Can you work these out from the model? Positions are in its coordinate system, mm. Face numbers are marked on the shaded views. Round coordinates to 2 decimals unless told otherwise and drop trailing zeros. Loops run counter-clockwise (first coordinate to the right, second up) from the corner with the lowest first, then second, coordinate; pieces in that order, holes last. Notation, with made-up numbers: M -2.75,-35 L 39.25,-35 A11 cw 39.25,-23 Z; hole C -8,45.25 d11. An arc over 180 degrees is marked long. Use a Markdown table: item, result. Add a question column.
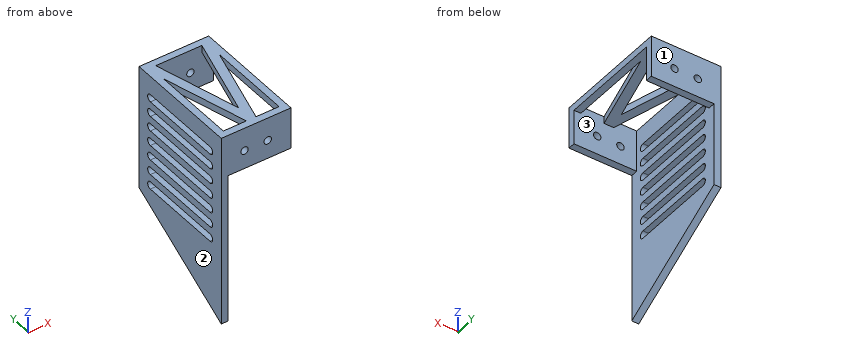
```python
from build123d import *

# Parameters (mm, degrees)
SKETCH_1_W      = 30
SKETCH_1_H      = 50
EXTRUDE_1_DEPTH = 3
EXTRUDE_3_DEPTH = 3
EXTRUDE_START   = -50
SKETCH_3_W      = 27
SKETCH_3_H      = 15
SKETCH_3_R      = 1.6
EXTRUDE_4_DEPTH = 3
SKETCH_5_W      = 27
SKETCH_5_H      = 15
SKETCH_5_R      = 1.6
EXTRUDE_5_DEPTH = 3


with BuildPart() as part:
    # 草图1 → 凸台-拉伸1 (new body)
    with BuildSketch(Plane.XY):
        with Locations((-1.547723223, -1.182673383)):
            Rectangle(SKETCH_1_W, SKETCH_1_H)
        Polygon((-13.547723223, 13.216157116), (-13.547723223, -23.182673383), (-3.620769451, -23.182673383), align=None, mode=Mode.SUBTRACT)
        Polygon((10.452276777, 13.216157116), (10.452276777, -23.182673383), (0.525323004, -23.182673383), align=None, mode=Mode.SUBTRACT)
        Polygon((-11.474676996, 20.817326617), (8.379230549, 20.817326617), (-1.547723223, -15.581503883), align=None, mode=Mode.SUBTRACT)
    extrude(amount=EXTRUDE_1_DEPTH)

    # 草图2 → 凸台-拉伸3 (add)
    with BuildSketch(Plane.ZY.offset(16.547723223)):
        Polygon((-80, -26.182673383), (-51.132486541, 23.817326617), (0, 23.817326617), (0, -26.182673383), align=None)
        Polygon((-3, -23.182673383), (-3, 20.817326617), (-49.400435733, 20.817326617), (-74.803847577, -23.182673383), align=None, mode=Mode.SUBTRACT)
        Polygon((-3, -23.182673383), (-74.803847577, -23.182673383), (-49.400435733, 20.817326617), (-3, 20.817326617), align=None)
        with BuildLine():
            ThreePointArc((-8.378224309, -19.337056165), (-6.74645341, -20.968827063), (-5.114682512, -19.337056165))
            Line((-5.114682512, -19.337056165), (-5.114682512, 16.93515829))
            ThreePointArc((-5.114682512, 16.93515829), (-6.74645341, 18.566929189), (-8.378224309, 16.93515829))
            Line((-8.378224309, 16.93515829), (-8.378224309, -19.337056165))
        make_face(mode=Mode.SUBTRACT)
        with BuildLine():
            ThreePointArc((-14.878224309, -19.337056165), (-13.24645341, -20.968827063), (-11.614682512, -19.337056165))
            Line((-11.614682512, -19.337056165), (-11.614682512, 16.93515829))
            ThreePointArc((-11.614682512, 16.93515829), (-13.24645341, 18.566929189), (-14.878224309, 16.93515829))
            Line((-14.878224309, 16.93515829), (-14.878224309, -19.337056165))
        make_face(mode=Mode.SUBTRACT)
        with BuildLine():
            ThreePointArc((-21.378224309, -19.337056165), (-19.74645341, -20.968827063), (-18.114682512, -19.337056165))
            Line((-18.114682512, -19.337056165), (-18.114682512, 16.93515829))
            ThreePointArc((-18.114682512, 16.93515829), (-19.74645341, 18.566929189), (-21.378224309, 16.93515829))
            Line((-21.378224309, 16.93515829), (-21.378224309, -19.337056165))
        make_face(mode=Mode.SUBTRACT)
        with BuildLine():
            ThreePointArc((-27.878224309, -19.337056165), (-26.24645341, -20.968827063), (-24.614682512, -19.337056165))
            Line((-24.614682512, -19.337056165), (-24.614682512, 16.93515829))
            ThreePointArc((-24.614682512, 16.93515829), (-26.24645341, 18.566929189), (-27.878224309, 16.93515829))
            Line((-27.878224309, 16.93515829), (-27.878224309, -19.337056165))
        make_face(mode=Mode.SUBTRACT)
        with BuildLine():
            ThreePointArc((-34.378224309, -19.337056165), (-32.74645341, -20.968827063), (-31.114682512, -19.337056165))
            Line((-31.114682512, -19.337056165), (-31.114682512, 16.93515829))
            ThreePointArc((-31.114682512, 16.93515829), (-32.74645341, 18.566929189), (-34.378224309, 16.93515829))
            Line((-34.378224309, 16.93515829), (-34.378224309, -19.337056165))
        make_face(mode=Mode.SUBTRACT)
        with BuildLine():
            ThreePointArc((-40.878224309, -19.337056165), (-39.24645341, -20.968827063), (-37.614682512, -19.337056165))
            Line((-37.614682512, -19.337056165), (-37.614682512, 16.93515829))
            ThreePointArc((-37.614682512, 16.93515829), (-39.24645341, 18.566929189), (-40.878224309, 16.93515829))
            Line((-40.878224309, 16.93515829), (-40.878224309, -19.337056165))
        make_face(mode=Mode.SUBTRACT)
        with BuildLine():
            ThreePointArc((-47.378224309, -19.337056165), (-45.74645341, -20.968827063), (-44.114682512, -19.337056165))
            Line((-44.114682512, -19.337056165), (-44.114682512, 16.93515829))
            ThreePointArc((-44.114682512, 16.93515829), (-45.74645341, 18.566929189), (-47.378224309, 16.93515829))
            Line((-47.378224309, 16.93515829), (-47.378224309, -19.337056165))
        make_face(mode=Mode.SUBTRACT)
    extrude(amount=-EXTRUDE_3_DEPTH)

    # 草图3 → 凸台-拉伸4 (add)
    with BuildSketch(Plane(origin=(0, 23.817326617, 0), x_dir=(1, 0, 0), z_dir=(0, 1, 0)).offset(EXTRUDE_START)):
        with Locations((-0.047723223, 7.5)):
            Rectangle(SKETCH_3_W, SKETCH_3_H)
        with Locations((-6.547723223, 7)):
            Circle(SKETCH_3_R, mode=Mode.SUBTRACT)
        with Locations((3.452276777, 7)):
            Circle(SKETCH_3_R, mode=Mode.SUBTRACT)
    extrude(amount=EXTRUDE_4_DEPTH)

    # 草图5 → 凸台-拉伸5 (add)
    with BuildSketch(Plane(origin=(0, 23.817326617, 0), x_dir=(1, 0, 0), z_dir=(0, 1, 0))):
        with Locations((-0.047723223, 7.5)):
            Rectangle(SKETCH_5_W, SKETCH_5_H)
        with Locations((-6.547723223, 7)):
            Circle(SKETCH_5_R, mode=Mode.SUBTRACT)
        with Locations((3.452276777, 7)):
            Circle(SKETCH_5_R, mode=Mode.SUBTRACT)
    extrude(amount=-EXTRUDE_5_DEPTH)


solid = part.part
```
(1) Thinking about a two-plate mould opening in Y: for the marked faces 1, 2 and 3, which applies, released by +Y, released by -Y, zero draft, split by the parting line, or undercut?
(2) Suppose I cut it at A-A on z = -39. List the corners of the cut face in (x, y) for me, and give its area (3 significant figures).
(3) I'm going to push flat-ended pins straight in: pin 1 (0.9 mm diameter, centred on x = -15, y = -2.5, fed in from -Z); pin 2 (4 mm diameter, centred on y = -20, z = -9.5, fed in from +X); pin 3 (3.5 mm diameter, centred on x = -15, y = -1, fed in from -Z). Where does each tip first touch, or does it pass through?
(4) If I drill on probe 1 along X at (y, z) = (22.25, -7); probe 2 along Y at (x, z) = (-5, -8.5); probe 3 along X at (y, z) = (-17.5, -44), over which ranges is the centre line in solid material (lowest first)? Write a range as [from, to].
(5) Suppose I cut it at D-D on y = -11.5. Count the separate pieces of the cut face and the enclosed holes in it, and give its area (3 significant figures).
(6) Suppose I cut it at C-C on x = 2.75. List the corners of the cut face in (y, z) for me.
(7) Suppose I cut it at B-B on z = -7. List the corners of the cut face in (x, y) for me, and give its area (3 significant figures).
Results below:
| question | item | result |
|---|---|---|
| 1 | face 1 | released by +Y |
| 1 | face 2 | zero draft |
| 1 | face 3 | undercut |
| 2 | outline | M -16.55,-26.18 L -13.55,-26.18 L -13.55,-20.95 L -16.55,-20.95 Z; M -16.55,18.55 L -13.55,18.55 L -13.55,23.82 L -16.55,23.82 Z |
| 2 | area | 31.5 mm² |
| 3 | pin 1 | stops at z = -66.59 |
| 3 | pin 2 | stops at x = -13.55 |
| 3 | pin 3 | stops at z = -66.47 |
| 4 | probe 1 | x = [-16.55, -8.15], [-4.95, 1.85], [5.05, 13.45] |
| 4 | probe 2 | y = [-26.18, -23.18], [20.82, 23.82] |
| 4 | probe 3 | x = [-16.55, -13.55] |
| 5 | separate pieces | 11 |
| 5 | enclosed holes | 0 |
| 5 | area | 189 mm² |
| 6 | outline | M -26.18,-15 L -23.18,-15 L -23.18,-8.44 L -26.18,-8.44 Z; M -26.18,-5.56 L -23.18,-5.56 L -23.18,3 L -26.18,3 Z; M -15.03,0 L 0.18,0 L 0.18,3 L -15.03,3 Z; M 20.82,-15 L 23.82,-15 L 23.82,-8.44 L 20.82,-8.44 Z; M 20.82,-5.56 L 23.82,-5.56 L 23.82,3 L 20.82,3 Z |
| 7 | outline | M -16.55,-26.18 L -8.15,-26.18 L -8.15,-23.18 L -13.55,-23.18 L -13.55,-20.95 L -16.55,-20.95 Z; M -16.55,18.55 L -13.55,18.55 L -13.55,20.82 L -8.15,20.82 L -8.15,23.82 L -16.55,23.82 Z; M -4.95,-26.18 L 1.85,-26.18 L 1.85,-23.18 L -4.95,-23.18 Z; M -4.95,20.82 L 1.85,20.82 L 1.85,23.82 L -4.95,23.82 Z; M 5.05,-26.18 L 13.45,-26.18 L 13.45,-23.18 L 5.05,-23.18 Z; M 5.05,20.82 L 13.45,20.82 L 13.45,23.82 L 5.05,23.82 Z |
| 7 | area | 155 mm² |
